from build123d import *

# Parameters (mm, degrees)
F0_W      = 25
F0_H      = 45
F1_DEPTH  = 2
F2_W      = 25
F2_H      = 45
F2_W_2    = 21
F2_H_2    = 41
F3_DEPTH  = 16
F4_R      = 5.75
F5_DEPTH  = 8
F6_R      = 3.75
F7_DEPTH  = 3
F8_R      = 3.5
F9_DEPTH  = 3
F10_R     = 5.25
F11_DEPTH = 3
F12_R     = 5.25
F13_DEPTH = 3
F14_R     = 3.75
F15_DEPTH = 6.5
F16_R     = 3.75
F17_DEPTH = 6.5
F18_R     = 1.25
F19_R     = 2.25
F20_DEPTH = 25
F21_R     = 2.25
F22_DEPTH = 25


with BuildPart() as f1:
    # F0 (on Front) → F1 (new body)
    with BuildSketch(Plane.XZ):
        Rectangle(F0_W, F0_H)
    extrude(amount=F1_DEPTH)

    # F2 (on face) → F3 (join)
    with BuildSketch(Plane.XZ.offset(2)):
        Rectangle(F2_W, F2_H)
        Rectangle(F2_W_2, F2_H_2, mode=Mode.SUBTRACT)
    extrude(amount=F3_DEPTH)

    # F4 (on face) → F5 (join)
    with BuildSketch(Plane.YZ.offset(12.5)):
        with Locations((-9.5, 12.75)):
            Circle(F4_R)
        with Locations((-9.5, -12.75)):
            Circle(F4_R)
    extrude(amount=F5_DEPTH)

    # F6 (on face) → F7 (join)
    with BuildSketch(Plane.YZ.offset(20.5)):
        with Locations((-9.5, 12.75)):
            Circle(F6_R)
    extrude(amount=F7_DEPTH)

    # F8 (on face) → F9 (join)
    with BuildSketch(Plane.YZ.offset(20.5)):
        with Locations((-9.5, -12.75)):
            Circle(F8_R)
    extrude(amount=F9_DEPTH)

    # F10 (on face) → F11 (join)
    with BuildSketch(Plane.YZ.offset(23.5)):
        with Locations((-9.5, 12.75)):
            Circle(F10_R)
    extrude(amount=F11_DEPTH)

    # F12 (on face) → F13 (join)
    with BuildSketch(Plane.YZ.offset(23.5)):
        with Locations((-9.5, -12.75)):
            Circle(F12_R)
    extrude(amount=F13_DEPTH)

    # F14 (on face) → F15 (join)
    with BuildSketch(Plane.YZ.offset(26.5)):
        with Locations((-9.5, 12.75)):
            Circle(F14_R)
    extrude(amount=F15_DEPTH)

    # F16 (on face) → F17 (join)
    with BuildSketch(Plane.YZ.offset(26.5)):
        with Locations((-9.5, -12.75)):
            Circle(F16_R)
    extrude(amount=F17_DEPTH)

    # F18
    f18_edges = [f1.edges().sort_by_distance(p)[0] for p in [
        (26.5, -14.75, 12.75),
        (26.5, -14.75, -12.75),
        (23.5, -14.75, -12.75),
        (23.5, -14.75, 12.75),
    ]]
    fillet(f18_edges, radius=F18_R)

    # F19 (on face) → F20 (cut)
    with BuildSketch(Plane.YZ.offset(33)):
        with Locations((-9.5, 12.75)):
            Circle(F19_R)
    extrude(amount=-F20_DEPTH, mode=Mode.SUBTRACT)

    # F21 (on face) → F22 (cut)
    with BuildSketch(Plane.YZ.offset(33)):
        with Locations((-9.5, -12.75)):
            Circle(F21_R)
    extrude(amount=-F22_DEPTH, mode=Mode.SUBTRACT)


solid = f1.part
CAD build for the part. Positions are in the model's coordinates, mm. A direction names the side the tool comes from. Coordinates: 2 decimals unless noted, no trailing zeros. Loops run counter-clockwise (first coordinate to the right, second up) from the corner with the lowest first, then second, coordinate; pieces in that order, holes last. Notation, with made-up numbers: (63, 71) - (81, 71) arc R21 cw to (81, 92) - close; hole circle Ø2 at (58.5, 64.5). An arc over 180 degrees is marked (long way). Write item = value, one per line. Start each with the question number.
Q1. Cut at B-B, the plane x = 4.5. List the corners of the cut face in (y, z), then the cut area to 3 significant figures.
Q2. Pull direction Z, two halves, no side cores. Call faces 1 (the flat face through (0, -10, -20.5)), 2 (the flat face through (0, -9, -22.5)), 3 (the flat face through (0, 0, 0)): pulls with the +Z half, pulls with the -Z half, needs draft (parallel to the pull), parting line crosses it, or undercut.
Q3. Cut at D-D, the plane z = -4. List the corners of the cut face in (x, y).
Q4. Which spindle directions (+Z, -Z, +X, -X, +Y, -Y) get a long thin tool onto all of the face, cutting with end or side? Do faces 4 (the flat face through (0, -9, 22.5)), 5 (the cylindrical face through (16.44, -6.41, -7.9)), 6 (the flat face through (-12.5, -9, 0)), 7 (the flat face through (0, -2, 0)), 8 (the cylindrical face through (21.979, -10.259, -16.167)). Say none if no direction does.
Q5. Drill centre lines: L1, parallel to Z at x = 23.25, y = -9.5; L2, parallel to Z at x = -3.5, y = -8.75; L3, parallel to X at y = -4, z = -4. Where is each one in solid material? Low to high.
Q6. Flat gauge pins, fed straight in: pin 1 Ø5 at (y, z) = (-4.5, -7.5) entering from +X; pin 2 Ø1 at (y, z) = (-8.5, -13.5) entering from +X; pin 3 Ø1.5 at (y, z) = (-3, -4.5) entering from +X. Where does each tip first touch, or does it go through?
Computed:
q1.outline = (-18, -22.5) - (0, -22.5) - (0, 22.5) - (-18, 22.5) - (-18, 20.5) - (-2, 20.5) - (-2, -20.5) - (-18, -20.5) - close
q1.area = 154 mm²
q2.face_1 = undercut
q2.face_2 = pulls with the -Z half
q2.face_3 = needs draft
q3.outline = (-12.5, -18) - (-10.5, -18) - (-10.5, -2) - (10.5, -2) - (10.5, -18) - (12.5, -18) - (12.5, 0) - (-12.5, 0) - close
q4.face_4 = +Z, +X, -X, +Y, -Y
q4.face_5 = +X
q4.face_6 = +Z, -Z, -X, +Y, -Y
q4.face_7 = -Y
q4.face_8 = none
q5.L1 = -16.25 to -15, -10.5 to -9.25, 9 to 10.5, 15 to 16.5
q5.L2 = -22.5 to -20.5, 20.5 to 22.5
q5.L3 = -12.5 to -10.5, 10.5 to 12.5
q6.pin_1 = 26.25
q6.pin_2 = -10.5
q6.pin_3 = 12.5
